The figure shows three views and two pictorial views of one solid part (mm, origin at its lowest corner). Answer the questions. A direction names the side the tool comes from. Coordinates: 2 decimals unless noted, no trailing zeros. Write each loop counter-clockwise with the first axis right and the second up, starting at its lowest first coordinate (ties: lowest second). Pieces come first, ordered by that corner, then holes. Notation, with made-up numbers: M 25.25,70.5 L 63.25,70.5 A25 ccw 63.25,107.5 Z; hole C 59,65 d11. An arc over 180 degrees is marked long. Write item = value, one per line. Start each with the question number.
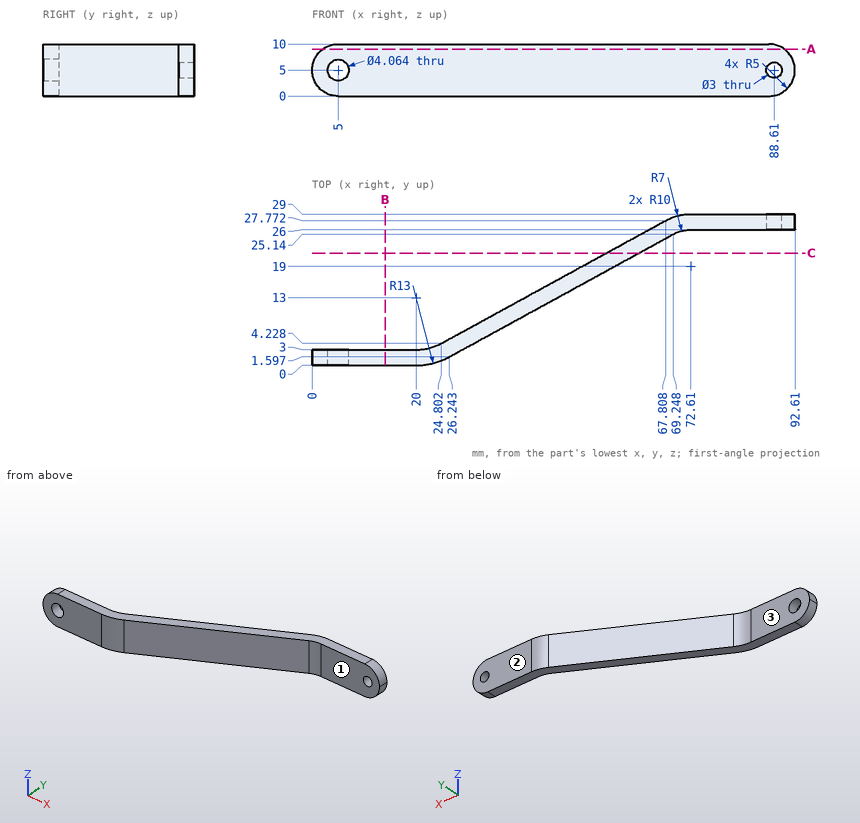
1. The part is cut by section B-B, the plane x = 14. Write down the section's boundary in (y, z).
2. For the marked faces 1, 2 and 3, determine the directions among +Z, -Z, +X, -X, +Y, -Y from which every point of the face is accessible in a straight line to the end or side of a thin tool.
3. The part is cut by section A-A, the plane z = 9. Write down the section's boundary in (x, y).
4. Straight lines are drawn through the part: L1, parallel to Y at x = 72.5, z = 9; L2, parallel to X at y = 1.7, z = 5 (1 decimal); L3, parallel to X at y = 1.2, z = 5 (1 decimal). For each, find the intervals that lie inside material, in ascending order. Write a range as [from, to].
5. Each of these flat-tipped pins is pushed along its axis until it touches: pin 1 (2 mm diameter, centred on x = 55, z = 6, fed in from +Y); pin 2 (5 mm diameter, centred on x = 12.5, z = 4, fed in from +Y); pin 3 (2.5 mm diameter, centred on x = 88.61, z = 5, fed in from +Y). Where does it stop, or does it pass through?
6. The part is cut by section C-C, the plane y = 21.5. Write down the section's boundary in (x, z).
Solution:
q1.outline = M 0,0 L 3,0 L 3,10 L 0,10 Z
q2.face_1 = +Z, -Z, +X, -Y
q2.face_2 = +Z, -Z, +X, -X, +Y
q2.face_3 = +Z, -Z, -X, +Y
q3.outline = M 2,0 L 20,0 A13 ccw 26.24,1.6 L 69.25,25.14 A7 cw 72.61,26 L 90.61,26 L 90.61,29 L 72.61,29 A10 ccw 67.81,27.77 L 24.8,4.23 A10 cw 20,3 L 2,3 Z
q4.L1 = [26, 29]
q4.L2 = [0, 3], [7, 26.4]
q4.L3 = [0, 3], [7, 25.5]
q5.pin_1 = 21.31
q5.pin_2 = 3
q5.pin_3 = through
q6.outline = M 56.35,0 L 62.6,0 L 62.6,10 L 56.35,10 Z
